from build123d import *

# Parameters (mm, degrees)
F0_W      = 125
F0_H      = 75
F1_DEPTH  = 23
F2_W      = 108
F2_H      = 65
F3_DEPTH  = 21
F4_W      = 8
F4_H      = 71
F5_DEPTH  = 21
F5_TAPER  = 3
F6_W      = 21
F6_H      = 71
F7_DEPTH  = 2.1
F8_W      = 108.9
F8_H      = 2
F9_DEPTH  = 2
F10_W     = 95
F10_H     = 2
F10_W_2   = 15
F11_DEPTH = 2
F12_R     = 2
F13_R     = 1
F14_R     = 1
F15_W     = 8
F15_H     = 1
F16_DEPTH = 2
F17_R     = 0.55
F18_DEPTH = 10.1
F19_R     = 0.55
F20_DEPTH = 10.1
F21_R     = 0.5
F22_DEPTH = 8
F23_W     = 5
F23_H     = 13
F24_DEPTH = 3


with BuildPart() as f1:
    # F0 (on Front) → F1 (new body)
    with BuildSketch(Plane.XZ):
        Rectangle(F0_W, F0_H)
    extrude(amount=F1_DEPTH)

    # F2 (on face) → F3 (cut)
    with BuildSketch(Plane.XZ.offset(23)):
        with Locations((6.5, 0)):
            Rectangle(F2_W, F2_H)
    extrude(amount=-F3_DEPTH, mode=Mode.SUBTRACT)

    # F4 (on face) → F5 (cut)
    with BuildSketch(Plane.XZ.offset(23)):
        with Locations((-56.5, 0)):
            Rectangle(F4_W, F4_H)
    extrude(amount=-F5_DEPTH, taper=F5_TAPER, mode=Mode.SUBTRACT)

    # F6 (on face) → F7 (cut)
    with BuildSketch(Plane.YZ.offset(62.5)):
        with Locations((-12.5, 0)):
            Rectangle(F6_W, F6_H)
    extrude(amount=-F7_DEPTH, mode=Mode.SUBTRACT)

    # F8 (on face) → F9 (cut)
    with BuildSketch(Plane.XZ.offset(23)):
        Polygon((-48.5, 33.5), (-50.5, 33.5), (-50.5, -35.5), (-48.5, -35.5), (-48.5, -33.5), align=None)
        Polygon((60.4, 33.5), (60.4, 35.5), (-50.5, 35.5), (-50.5, 33.5), (-48.5, 33.5), align=None)
        with Locations((5.95, -34.5)):
            Rectangle(F8_W, F8_H)
    extrude(amount=-F9_DEPTH, mode=Mode.SUBTRACT)

    # F10 (on face) → F11 (join)
    with BuildSketch(Plane.XZ.offset(2)):
        Rectangle(F10_W, F10_H)
        with Locations((55, 0)):
            Rectangle(F10_W_2, F10_H)
    extrude(amount=F11_DEPTH)

    # F12
    f12_edges = [f1.edges().sort_by_distance(p)[0] for p in [
        (62.5, -4, 0),
    ]]
    fillet(f12_edges, radius=F12_R)

    # F13
    f13_edges = [f1.edges().sort_by_distance(p)[0] for p in [
        (60.4, -12.5, 32.5),
        (60.4, -12.5, -32.5),
    ]]
    fillet(f13_edges, radius=F13_R)

    # F14
    f14_edges = [f1.edges().sort_by_distance(p)[0] for p in [
        (62.5, -11.5, -37.5),
        (62.5, 0, 0),
        (0, 0, -37.5),
        (62.5, -11.5, 37.5),
        (0, 0, 37.5),
        (-62.5, -11.5, 37.5),
        (-62.5, 0, 0),
        (-62.5, -11.5, -37.5),
    ]]
    fillet(f14_edges, radius=F14_R)

    # F15 (on face) → F16 (cut)
    with BuildSketch(Plane.XZ.offset(23)):
        with Locations((-56.5, 36)):
            Rectangle(F15_W, F15_H)
        Polygon((-60.5, -35.5), (-60.5, 35.5), (-60.5, 36.5), (-61.5, 36.5), (-61.5, -36.5), (-60.5, -36.5), align=None)
        Polygon((-52.5, 36.5), (-52.5, 35.5), (-52.5, -35.5), (-52.5, -36.5), (-51.5, -36.5), (-51.5, 36.5), align=None)
        with Locations((-56.5, -36)):
            Rectangle(F15_W, F15_H)
    extrude(amount=-F16_DEPTH, mode=Mode.SUBTRACT)

    # F17 (on face) → F18 (cut)
    with BuildSketch(Plane.YZ.offset(60.4)):
        with Locations((-19.5, -34.5)):
            Circle(F17_R)
        with Locations((-15.5, -34.5)):
            Circle(F17_R)
        with Locations((-11.5, -34.5)):
            Circle(F17_R)
        with Locations((-3.5, -34.5)):
            Circle(F17_R)
        with Locations((-7.5, -34.5)):
            Circle(F17_R)
    extrude(amount=-F18_DEPTH, mode=Mode.SUBTRACT)

    # F19 (on face) → F20 (cut)
    with BuildSketch(Plane.YZ.offset(60.4)):
        with Locations((-19.5, 34.5)):
            Circle(F19_R)
        with Locations((-15.5, 34.5)):
            Circle(F19_R)
        with Locations((-11.5, 34.5)):
            Circle(F19_R)
        with Locations((-7.5, 34.5)):
            Circle(F19_R)
        with Locations((-3.5, 34.5)):
            Circle(F19_R)
    extrude(amount=-F20_DEPTH, mode=Mode.SUBTRACT)

    # F21 (on face) → F22 (cut)
    with BuildSketch(Plane.YZ.offset(-47.5)):
        with Locations((-6, -28.5)):
            Circle(F21_R)
        with Locations((-6, 28.5)):
            Circle(F21_R)
    extrude(amount=-F22_DEPTH, mode=Mode.SUBTRACT)

    # F23 (on face) → F24 (cut)
    with BuildSketch(Plane.XY.offset(37.5)):
        with Locations((-56, -12.5)):
            Rectangle(F23_W, F23_H)
    extrude(amount=-F24_DEPTH, mode=Mode.SUBTRACT)


solid = f1.part
Design review of the part built by this model. Coordinates are the model's own, in mm. A direction names the side the tool comes from. Round coordinates to 2 decimals unless told otherwise and drop trailing zeros. Write each loop counter-clockwise with the first axis right and the second up, starting at its lowest first coordinate (ties: lowest second). Pieces come first, ordered by that corner, then holes.
Item 1: Wall thickness on L1, parallel to Z at x = 53.25, y = -19.5; L2, parallel to Y at x = 55.5, z = 34.5; L3, parallel to Z at x = -37.5, y = -21.5: over which ranges is each line inside the solid? List them lowest first.
Item 2: For faces 1 (the flat face through (-57, -2, 0)), 2 (the flat face through (-58.5, -13, 36)), 3 (the flat face through (5, -13, 32.5)), list the 3-axis set-ups (+Z, -Z, +X, -X, +Y, -Y) from which the entire face can be reached by the end or side of a thin tool; tool diameter is ignored.
Item 3: Consider section A-A on x = -5.5. Give the boundary of the cut face in (y, z).
Item 4: Draft analysis for pull direction X (two halves, no side actions). For faces 4 (the flat face through (-1, 0, 1)), 5 (the flat face through (62.5, -1.4, -0.2)), 6 (the flat face through (-52, -21, 0)), state which applies: released by +X, released by -X, zero draft, split by the parting line, or undercut.
Item 5: For pin 1 Ø12 at (y, z) = (-15.5, 14) entering from +X; pin 2 Ø0.9 at (y, z) = (-11.5, 34.5) entering from +X; pin 3 Ø1.3 at (y, z) = (-11.5, -34.5) entering from +X, all flat-tipped, find the tip position at first contact; note any pin that passes through.
Check values:
1. L1: z = -37.5 to -35.05, -33.95 to -32.5, 32.5 to 33.95, 35.05 to 37.5
1. L2: y = -21 to -20.05, -18.95 to -16.05, -14.95 to -12.05, -10.95 to -8.05, -6.95 to -4.05, -2.95 to 0
1. L3: z = -37.5 to -35.5, -33.5 to -32.5, 32.5 to 33.5, 35.5 to 37.5
2. face 1: -Y
2. face 2: +Z
2. face 3: +X, -Y
3. outline: (-23, -37.5) - (-1, -37.5) arc R1 ccw to (0, -36.5) - (0, 36.5) arc R1 ccw to (-1, 37.5) - (-23, 37.5) - (-23, 35.5) - (-21, 35.5) - (-21, 33.5) - (-23, 33.5) - (-23, 32.5) - (-2, 32.5) - (-2, 1) - (-4, 1) - (-4, -1) - (-2, -1) - (-2, -32.5) - (-23, -32.5) - (-23, -33.5) - (-21, -33.5) - (-21, -35.5) - (-23, -35.5) - close
4. face 4: zero draft
4. face 5: released by +X
4. face 6: undercut
5. pin 1: stops at x = -47.5
5. pin 2: stops at x = 50.3
5. pin 3: stops at x = 60.4
